```python
from build123d import *

# Parameters (mm, degrees)
BOSS_EXTRUDE1_DEPTH = 4
SKETCH3_R           = 3
CUT_EXTRUDE1_DEPTH  = 5


with BuildPart() as part:
    # Sketch2 → Boss-Extrude1 (new body)
    with BuildSketch(Plane(origin=(0, 0, 0), x_dir=(1, 0, 0), z_dir=(0, 1, 0))):
        Polygon((0, 0), (0, 60), (20, 60), (60, 20), (60, 0), align=None)
    extrude(amount=BOSS_EXTRUDE1_DEPTH)

    # Sketch3 → Cut-Extrude1 (cut, through all)
    with BuildSketch(Plane(origin=(0, 4, 0), x_dir=(1, 0, 0), z_dir=(0, 1, 0))):
        with Locations((10, 10)):
            Circle(SKETCH3_R)
        with Locations((30, 10)):
            Circle(SKETCH3_R)
        with Locations((50, 10)):
            Circle(SKETCH3_R)
        with Locations((10, 50)):
            Circle(SKETCH3_R)
        with Locations((10, 30)):
            Circle(SKETCH3_R)
    extrude(amount=-CUT_EXTRUDE1_DEPTH, mode=Mode.SUBTRACT)


solid = part.part
```
Design review of the part built by this model. Coordinates are the model's own, in mm. Round coordinates to 2 decimals unless told otherwise and drop trailing zeros. Write each loop counter-clockwise with the first axis right and the second up, starting at its lowest first coordinate (ties: lowest second). Pieces come first, ordered by that corner, then holes. Notation, with made-up numbers: (72.25, 53) -> (101.25, 53) arc R24 cw to (101.25, 86) -> close; hole circle Ø1 at (5, 75.25). An arc over 180 degrees is marked (long way). Answer in a Markdown table with one row per item.
Q1. Take a section at C-C, the plane z = -10. State the section outline as (x, y) points.
The answers:
| item | result |
|---|---|
| outline | (0, 0) -> (7, 0) -> (7, 4) -> (0, 4) -> close; (13, 0) -> (27, 0) -> (27, 4) -> (13, 4) -> close; (33, 0) -> (47, 0) -> (47, 4) -> (33, 4) -> close; (53, 0) -> (60, 0) -> (60, 4) -> (53, 4) -> close |
Q2. Take a section at A-A, the plane z = -30. State the section outline as (x, y) points, then the cut area to 3 significant figures.
The answers:
| item | result |
|---|---|
| outline | (0, 0) -> (7, 0) -> (7, 4) -> (0, 4) -> close; (13, 0) -> (50, 0) -> (50, 4) -> (13, 4) -> close |
| area | 176 mm² |
Q3. Draft analysis for pull direction X (two halves, no side actions). For faces 1 (the face through (10, 2, -60)), 2 (the face through (0, 2, -30)), 3 (the face through (12.77, 2.03, -8.85)), state which applies: +X half, -X half, draft (parallel to the pull), parting line (faces both ways), or undercut.
The answers:
| item | result |
|---|---|
| face 1 | draft |
| face 2 | -X half |
| face 3 | undercut |
Q4. Take a section at D-D, the plane x = 10. State the section outline as (y, z) points.
The answers:
| item | result |
|---|---|
| outline | (0, -60) -> (4, -60) -> (4, -53) -> (0, -53) -> close; (0, -47) -> (4, -47) -> (4, -33) -> (0, -33) -> close; (0, -27) -> (4, -27) -> (4, -13) -> (0, -13) -> close; (0, -7) -> (4, -7) -> (4, 0) -> (0, 0) -> close |
Q5. To check wall thickness, follow L1, parallel to X at y = 2.2, z = -10; L2, parallel to Z at x = 10, y = 2.6; L3, parallel to Z at x = 8, y = 0.85. State the ranges of each line that lie inside material, in increasing order. Write a range as [from, to].
The answers:
| item | result |
|---|---|
| L1 | [0, 7], [13, 27], [33, 47], [53, 60] |
| L2 | [-60, -53], [-47, -33], [-27, -13], [-7, 0] |
| L3 | [-60, -52.24], [-47.76, -32.24], [-27.76, -12.24], [-7.76, 0] |
Q6. Clearance check with a flat-ended pin moving along its axis: pin 1 Ø3.5 at (x, z) = (10, -50) entering from -Y. State where the tip first meets the part, or that it passes through.
The answers:
| item | result |
|---|---|
| pin 1 | through |
Q7. Take a section at B-B, the plane x = 30. State the section outline as (y, z) points.
The answers:
| item | result |
|---|---|
| outline | (0, -50) -> (4, -50) -> (4, -13) -> (0, -13) -> close; (0, -7) -> (4, -7) -> (4, 0) -> (0, 0) -> close |
